Autodesk Inventor part; units mm, degrees
ref_plane "CS_ANBAU_HINTEN_LINKS_XY" through (161, 0, 20) normal (1, 0, 0) x (0, 0, -1)
ref_plane "CS_ANBAU_HINTEN_LINKS_YZ" through (161, 0, 20) normal (0, 0, -1) x (0, 1, 0)
ref_plane "CS_ANBAU_HINTEN_LINKS_ZX" through (161, 0, 20) normal (0, 1, 0) x (1, 0, 0)
sketch "Skizze_1" plane through (0, 0, 0) normal (1, 0, 0) x (0, 1, 0)
  line L0 (18.75, 20) -> (7, 20)
  line L1 (7, 20) -> (7, 15.5)
  line L2 (7, 15.5) -> (11.7, 15.5)
  line L3 (11.7, 15.5) -> (11.7, 13.82)
  line L4 (11.7, 13.82) -> (6.4481, 8.5681)
  line L5 (6.4481, 8.5681) -> (2, 6)
  line L6 (2, 6) -> (-2, 6)
  line L7 (-2, 6) -> (-6.4481, 8.5681)
  line L8 (-6.4481, 8.5681) -> (-11.7, 13.82)
  line L9 (-11.7, 13.82) -> (-11.7, 15.5)
  line L10 (-11.7, 15.5) -> (-7, 15.5)
  line L11 (-7, 15.5) -> (-7, 20)
  line L12 (-7, 20) -> (-18.75, 20)
  line L13 (-18.75, 20) -> (-20, 18.75)
  line L14 (-20, 18.75) -> (-20, 7)
  line L15 (-20, 7) -> (-15.5, 7)
  line L16 (-15.5, 7) -> (-15.5, 11.7)
  line L17 (-15.5, 11.7) -> (-13.82, 11.7)
  line L18 (-13.82, 11.7) -> (-8.5681, 6.4481)
  line L19 (-8.5681, 6.4481) -> (-6, 2)
  line L20 (-6, 2) -> (-6, -2)
  line L21 (-6, -2) -> (-8.5681, -6.4481)
  line L22 (-8.5681, -6.4481) -> (-13.82, -11.7)
  line L23 (-13.82, -11.7) -> (-15.5, -11.7)
  line L24 (-15.5, -11.7) -> (-15.5, -7)
  line L25 (-15.5, -7) -> (-20, -7)
  line L26 (-20, -7) -> (-20, -18.75)
  line L27 (-20, -18.75) -> (-18.75, -20)
  line L28 (-18.75, -20) -> (-7, -20)
  line L29 (-7, -20) -> (-7, -15.5)
  line L30 (-7, -15.5) -> (-11.7, -15.5)
  line L31 (-11.7, -15.5) -> (-11.7, -13.82)
  line L32 (-11.7, -13.82) -> (-6.4481, -8.5681)
  line L33 (-6.4481, -8.5681) -> (-2, -6)
  line L34 (-2, -6) -> (2, -6)
  line L35 (2, -6) -> (6.4481, -8.5681)
  line L36 (6.4481, -8.5681) -> (11.7, -13.82)
  line L37 (11.7, -13.82) -> (11.7, -15.5)
  line L38 (11.7, -15.5) -> (7, -15.5)
  line L39 (7, -15.5) -> (7, -20)
  line L40 (7, -20) -> (18.75, -20)
  line L41 (18.75, -20) -> (20, -18.75)
  line L42 (20, -18.75) -> (20, -7)
  line L43 (20, -7) -> (15.5, -7)
  line L44 (15.5, -7) -> (15.5, -11.7)
  line L45 (15.5, -11.7) -> (13.82, -11.7)
  line L46 (13.82, -11.7) -> (8.5681, -6.4481)
  line L47 (8.5681, -6.4481) -> (6, -2)
  line L48 (6, -2) -> (6, 2)
  line L49 (6, 2) -> (8.5681, 6.4481)
  line L50 (8.5681, 6.4481) -> (13.82, 11.7)
  line L51 (13.82, 11.7) -> (15.5, 11.7)
  line L52 (15.5, 11.7) -> (15.5, 7)
  line L53 (15.5, 7) -> (20, 7)
  line L54 (20, 7) -> (20, 18.75)
  line L55 (20, 18.75) -> (18.75, 20)
  line L56 (17.75, -12.1) -> (17.1, -12.1)
  line L57 (17.1, -12.1) -> (15.45, -13.75)
  line L58 (15.45, -13.75) -> (14.5, -13.75)
  arc A0 (14.5, -13.75) -> (13.75, -14.5) centre (14.5, -14.5) ccw
  line L59 (13.75, -14.5) -> (13.75, -15.45)
  line L60 (13.75, -15.45) -> (12.1, -17.1)
  line L61 (12.1, -17.1) -> (12.1, -17.75)
  arc A1 (12.1, -17.75) -> (12.85, -18.5) centre (12.85, -17.75) ccw
  line L62 (12.85, -18.5) -> (17.5, -18.5)
  arc A2 (17.5, -18.5) -> (18.5, -17.5) centre (17.5, -17.5) ccw
  line L63 (18.5, -17.5) -> (18.5, -12.85)
  arc A3 (18.5, -12.85) -> (17.75, -12.1) centre (17.75, -12.85) ccw
  line L64 (-17.1, -12.1) -> (-17.75, -12.1)
  arc A4 (-17.75, -12.1) -> (-18.5, -12.85) centre (-17.75, -12.85) ccw
  line L65 (-18.5, -12.85) -> (-18.5, -17.5)
  arc A5 (-18.5, -17.5) -> (-17.5, -18.5) centre (-17.5, -17.5) ccw
  line L66 (-17.5, -18.5) -> (-12.85, -18.5)
  arc A6 (-12.85, -18.5) -> (-12.1, -17.75) centre (-12.85, -17.75) ccw
  line L67 (-12.1, -17.75) -> (-12.1, -17.1)
  line L68 (-12.1, -17.1) -> (-13.75, -15.45)
  line L69 (-13.75, -15.45) -> (-13.75, -14.5)
  arc A7 (-13.75, -14.5) -> (-14.5, -13.75) centre (-14.5, -14.5) ccw
  line L70 (-14.5, -13.75) -> (-15.45, -13.75)
  line L71 (-15.45, -13.75) -> (-17.1, -12.1)
  circle A8 centre (0, 0) radius 3.5
  arc A9 (-17.5, 18.5) -> (-18.5, 17.5) centre (-17.5, 17.5) ccw
  line L72 (-18.5, 17.5) -> (-18.5, 12.85)
  arc A10 (-18.5, 12.85) -> (-17.75, 12.1) centre (-17.75, 12.85) ccw
  line L73 (-17.75, 12.1) -> (-17.1, 12.1)
  line L74 (-17.1, 12.1) -> (-15.45, 13.75)
  line L75 (-15.45, 13.75) -> (-14.5, 13.75)
  arc A11 (-14.5, 13.75) -> (-13.75, 14.5) centre (-14.5, 14.5) ccw
  line L76 (-13.75, 14.5) -> (-13.75, 15.45)
  line L77 (-13.75, 15.45) -> (-12.1, 17.1)
  line L78 (-12.1, 17.1) -> (-12.1, 17.75)
  arc A12 (-12.1, 17.75) -> (-12.85, 18.5) centre (-12.85, 17.75) ccw
  line L79 (-12.85, 18.5) -> (-17.5, 18.5)
  line L80 (17.5, 18.5) -> (12.85, 18.5)
  arc A13 (12.85, 18.5) -> (12.1, 17.75) centre (12.85, 17.75) ccw
  line L81 (12.1, 17.75) -> (12.1, 17.1)
  line L82 (12.1, 17.1) -> (13.75, 15.45)
  line L83 (13.75, 15.45) -> (13.75, 14.5)
  arc A14 (13.75, 14.5) -> (14.5, 13.75) centre (14.5, 14.5) ccw
  line L84 (14.5, 13.75) -> (15.45, 13.75)
  line L85 (15.45, 13.75) -> (17.1, 12.1)
  line L86 (17.1, 12.1) -> (17.75, 12.1)
  arc A15 (17.75, 12.1) -> (18.5, 12.85) centre (17.75, 12.85) ccw
  line L87 (18.5, 12.85) -> (18.5, 17.5)
  arc A16 (18.5, 17.5) -> (17.5, 18.5) centre (17.5, 17.5) ccw
extrude "Extrusion1" add sketch "Skizze_1" along normal blind 161
ref_plane "CS_ANBAU_HINTEN_LINKS_XY" through (161, 0, 20) normal (1, 0, 0) x (0, 0, -1)
ref_plane "CS_ANBAU_HINTEN_LINKS_YZ" through (161, 0, 20) normal (0, 0, -1) x (0, 1, 0)
ref_plane "CS_ANBAU_HINTEN_LINKS_ZX" through (161, 0, 20) normal (0, 1, 0) x (1, 0, 0)
ref_plane "CS_ANBAU_HINTEN_OBEN_XY" through (161, 20, 0) normal (1, 0, 0) x (0, 0, -1)
ref_plane "CS_ANBAU_HINTEN_OBEN_YZ" through (161, 20, 0) normal (0, 0, -1) x (0, 1, 0)
ref_plane "CS_ANBAU_HINTEN_OBEN_ZX" through (161, 20, 0) normal (0, 1, 0) x (1, 0, 0)
ref_plane "CS_ANBAU_HINTEN_RECHTS_XY" through (161, 0, -20) normal (1, 0, 0) x (0, 0, -1)
ref_plane "CS_ANBAU_HINTEN_RECHTS_YZ" through (161, 0, -20) normal (0, 0, -1) x (0, 1, 0)
ref_plane "CS_ANBAU_HINTEN_RECHTS_ZX" through (161, 0, -20) normal (0, 1, 0) x (1, 0, 0)
ref_plane "CS_ANBAU_HINTEN_UNTEN_XY" through (161, -20, 0) normal (1, 0, 0) x (0, 0, -1)
ref_plane "CS_ANBAU_HINTEN_UNTEN_YZ" through (161, -20, 0) normal (0, 0, -1) x (0, 1, 0)
ref_plane "CS_ANBAU_HINTEN_UNTEN_ZX" through (161, -20, 0) normal (0, 1, 0) x (1, 0, 0)
ref_plane "CS_ANBAU_QUER_XY" through (0, 0, 20) normal (0, 0, 1) x (1, 0, 0)
ref_plane "CS_ANBAU_QUER_YZ" through (0, 0, 20) normal (1, 0, 0) x (0, 1, 0)
ref_plane "CS_ANBAU_QUER_ZX" through (0, 0, 20) normal (0, 1, 0) x (0, 0, 1)
ref_plane "CS_ANBAU_QUER_1_XY" through (161, 0, 20) normal (0, 0, 1) x (1, 0, 0)
ref_plane "CS_ANBAU_QUER_1_YZ" through (161, 0, 20) normal (1, 0, 0) x (0, 1, 0)
ref_plane "CS_ANBAU_QUER_1_ZX" through (161, 0, 20) normal (0, 1, 0) x (0, 0, 1)
ref_plane "CS_ANBAU_VORNE_LINKS_XY" through (0, 0, 20) normal (-1, 0, 0) x (0, 0, -1)
ref_plane "CS_ANBAU_VORNE_LINKS_YZ" through (0, 0, 20) normal (0, 0, -1) x (0, -1, 0)
ref_plane "CS_ANBAU_VORNE_LINKS_ZX" through (0, 0, 20) normal (0, -1, 0) x (-1, 0, 0)
ref_plane "CS_ANBAU_VORNE_OBEN_XY" through (0, 20, 0) normal (-1, 0, 0) x (0, 0, -1)
ref_plane "CS_ANBAU_VORNE_OBEN_YZ" through (0, 20, 0) normal (0, 0, -1) x (0, -1, 0)
ref_plane "CS_ANBAU_VORNE_OBEN_ZX" through (0, 20, 0) normal (0, -1, 0) x (-1, 0, 0)
ref_plane "CS_ANBAU_VORNE_RECHTS_XY" through (0, 0, -20) normal (-1, 0, 0) x (0, 0, -1)
ref_plane "CS_ANBAU_VORNE_RECHTS_YZ" through (0, 0, -20) normal (0, 0, -1) x (0, -1, 0)
ref_plane "CS_ANBAU_VORNE_RECHTS_ZX" through (0, 0, -20) normal (0, -1, 0) x (-1, 0, 0)
ref_plane "CS_ANBAU_VORNE_UNTEN_XY" through (0, -20, 0) normal (-1, 0, 0) x (0, 0, -1)
ref_plane "CS_ANBAU_VORNE_UNTEN_YZ" through (0, -20, 0) normal (0, 0, -1) x (0, -1, 0)
ref_plane "CS_ANBAU_VORNE_UNTEN_ZX" through (0, -20, 0) normal (0, -1, 0) x (-1, 0, 0)
ref_plane "p1_XY" through (0, 20, 0) normal (0, 0, 1) x (1, 0, 0)
ref_plane "p1_YZ" through (0, 20, 0) normal (1, 0, 0) x (0, 1, 0)
ref_plane "p1_ZX" through (0, 20, 0) normal (0, 1, 0) x (0, 0, 1)
ref_plane "p2_XY" through (161, 20, 0) normal (0, 0, 1) x (1, 0, 0)
ref_plane "p2_YZ" through (161, 20, 0) normal (1, 0, 0) x (0, 1, 0)
ref_plane "p2_ZX" through (161, 20, 0) normal (0, 1, 0) x (0, 0, 1)
ref_plane "p3_XY" through (161, -20, 18.75) normal (1, 0, 0) x (0, 0, -1)
ref_plane "p3_YZ" through (161, -20, 18.75) normal (0, 0, -1) x (0, 1, 0)
ref_plane "p3_ZX" through (161, -20, 18.75) normal (0, 1, 0) x (1, 0, 0)
ref_plane "p4_XY" through (161, 20, 18.75) normal (1, 0, 0) x (0, 0, -1)
ref_plane "p4_YZ" through (161, 20, 18.75) normal (0, 0, -1) x (0, 1, 0)
ref_plane "p4_ZX" through (161, 20, 18.75) normal (0, 1, 0) x (1, 0, 0)
ref_plane "p5_XY" through (161, 20, -21.25) normal (1, 0, 0) x (0, 0, -1)
ref_plane "p5_YZ" through (161, 20, -21.25) normal (0, 0, -1) x (0, 1, 0)
ref_plane "p5_ZX" through (161, 20, -21.25) normal (0, 1, 0) x (1, 0, 0)
ref_plane "pm1_XY" through (0, 0, 0) normal (1, 0, 0) x (0, 0, -1)
ref_plane "pm1_YZ" through (0, 0, 0) normal (0, 0, -1) x (0, 1, 0)
ref_plane "pm1_ZX" through (0, 0, 0) normal (0, 1, 0) x (1, 0, 0)
ref_plane "pm2_XY" through (161, 0, -1.25) normal (1, 0, 0) x (0, 0, -1)
ref_plane "pm2_YZ" through (161, 0, -1.25) normal (0, 0, -1) x (0, 1, 0)
ref_plane "pm2_ZX" through (161, 0, -1.25) normal (0, 1, 0) x (1, 0, 0)
properties part number "Robotunits Profil 40 x 40 - PIL 4040 SNN 0161"
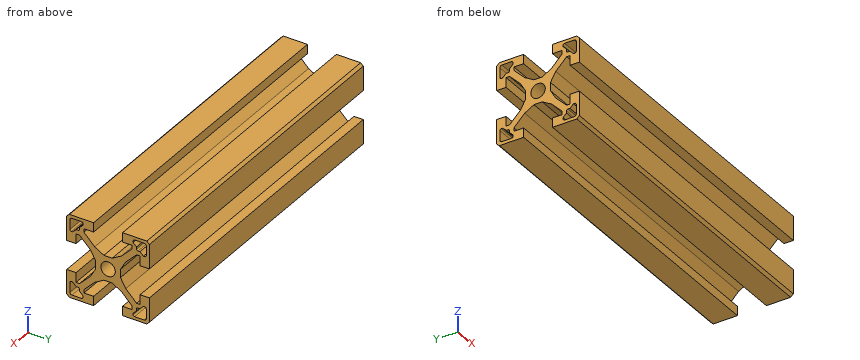
Verification items for the finished model (mm, model axes). Round coordinates to 2 decimals unless told otherwise and drop trailing zeros. Order: outer loops, then holes, each group sorted by start corner. A loop starts at its lowest first (then second) coordinate and runs counter-clockwise, first axis right, second up.
1. Section check A-A on z = 0. Record the cut outline in (x, y).
Final values:
outline: (0, -6) - (161, -6) - (161, -3.5) - (0, -3.5) - close; (0, 3.5) - (161, 3.5) - (161, 6) - (0, 6) - close
2. Section check C-C on x = 102. State how many separate pieces and enclosed holes the cut face has, then the cut area to 3 significant figures.
Final values:
separate pieces: 1
enclosed holes: 5
area: 564 mm2
3. Thickness scan on L1, parallel to Z at x = 71, y = 10.5; L2, parallel to Z at x = 89.5, y = 0; L3, parallel to Z at x = 60, y = 13. Record the ranges inside material, lowest first.
Final values:
L1: z = -20 to -15.5, -12.62 to -8.38, 8.38 to 12.62, 15.5 to 20
L2: z = -6 to -3.5, 3.5 to 6
L3: z = -20 to -18.5, -16.2 to -10.88, 10.88 to 16.2, 18.5 to 20
4. Go/stop test with flat-tipped pins: P1, Ø4.5, axis at x = 75, y = 1, coming from the +Z side; P2, Ø1.5, axis at y = 8, z = 11.5, coming from the +X side. Record where each tip stops, or that it passes through.
Final values:
P1: stops at z = 6.72
P2: passes through
